Could you check a few things on this model? Use its own coordinates, in mm. A direction names the side the tool comes from. Give positions to 0.01 mm unless a question says otherwise; leave off trailing zeros. Order: outer loops, then holes, each group sorted by start corner. A loop starts at its lowest first (then second) coordinate and runs counter-clockwise, first axis right, second up.
(1) Imagine slicing it at B-B, the plane x = -42. Write out the boundary of the cut face in (y, z), then the cut area to 3 significant figures.
(2) If we mould it in two halves opening along X, with no side actions, what happens to faces 1 (the flat face through (-37.26, 20.76, -6.14)), 2 (the cylindrical face through (-44.22, 28.83, -6.03)), 3 (the flat face through (-54.102, 29, -6)), 4 (the flat face through (-44, 28, -14.719))? For each: released by +X, released by -X, zero draft, split by the parting line, or undercut.
(3) Imagine slicing it at A-A, the plane z = -4. Write out the boundary of the cut face in (x, y).
(4) Will these pins go through, and if not, where does the flat tip stop? pin 1 (7.5 mm diameter, centred on x = -45.5, y = 20.5, fed in from +Z); pin 2 (8 mm diameter, centred on y = 23, z = -11, fed in from +X); pin 3 (3 mm diameter, centred on x = -63.5, y = 9.5, fed in from -Z); pin 4 (1.5 mm diameter, centred on x = -26, z = -11, fed in from -Y).
(5) Imagine slicing it at D-D, the plane y = 7.5. Write out the boundary of the cut face in (x, z).
(6) If I drill on probe 1 along Z at (x, y) = (-51.5, 4.5); probe 2 along Y at (x, z) = (-10.5, -7.5); probe 3 along Y at (x, z) = (-52, -9), over which ranges is the centre line in solid material (lowest first)?
(7) On a 3-axis mill with a long thin cutter (end or side, diameter ignored), from which of +Z, -Z, +X, -X, +Y, -Y can I reach the whole of each face in a straight line? I mean faces 5 (the flat face through (-44, 18, -5.512)), 6 (the flat face through (-44, 18, -6.782)), 7 (the flat face through (-45, 5, -12.294)), 8 (the flat face through (-34.036, 29, -6)). Say none if no direction works.
(8) Imagine slicing it at C-C, the plane y = 15. Write out the boundary of the cut face in (x, z).
Autodesk Inventor part; units mm, degrees
ref_plane "YZ Plane" through (0, 0, 0) normal (1, 0, 0) x (0, 1, 0)
ref_plane "XZ Plane" through (0, 0, 0) normal (0, 1, 0) x (-1, 0, 0)
ref_plane "XY Plane" through (0, 0, 0) normal (0, 0, 1) x (1, 0, 0)
sketch "Sketch1" plane through (0, 0, 0) normal (0, 1, 0) x (-1, 0, 0)
  line L0 (0, 0) -> (88.138, 0)
  line L1 (88.138, 0) -> (88.138, -12.2936)
  line L2 (88.138, -12.2936) -> (0, -12.2936)
  line L3 (0, -12.2936) -> (0, 0)
  dimension "d0" = 88.138
  dimension "d1" = 12.2936
extrude "Extrusion1" add sketch "Sketch1" along normal blind 10.922
sketch "Sketch2" plane through (0, 10.922, 0) normal (0, 1, 0) x (1, 0, 0)
  line L0 (-88.138, 12.2936) -> (-88.138, 0)
  line L1 (0, 0) -> (0, 12.2936)
  line L2 (-50.038, 6.7818) -> (-38.1, 6.7818)
  line L3 (-38.1, 6.7818) -> (-38.1, 5.5118)
  line L4 (-38.1, 5.5118) -> (-50.038, 5.5118)
  line L5 (-50.038, 5.5118) -> (-50.038, 6.7818)
  dimension "d7" = 11.938
  dimension "d8" = 1.27
extrude "Extrusion2" add sketch "Sketch2" along normal blind 5.08
sketch "Sketch4" plane through (-50.038, 10.922, -5.5118) normal (0, 0, 1) x (1, 0, 0)
  line L0 (0, 5.08) -> (11.938, 5.08)
  line L1 (11.938, 5.08) -> (0, 5.08)
  line L2 (11.938, 5.08) -> (13.6399, 14.732)
  line L3 (11.938, 5.08) -> (21.7389, 5.08) construction
  line L4 (0, 5.08) -> (-1.7019, 14.732)
  line L5 (0, 5.08) -> (9.8009, 5.08) construction
  line L6 (-1.7019, 14.732) -> (13.6399, 14.732)
  point P0 (50.038, -10.922)
  dimension "d12" = 80
  dimension "d13" = 100
extrude "Extrusion3" add sketch "Sketch4" against normal blind 1.27
sketch "Sketch5" plane through (-51.7399, 25.654, -5.5118) normal (0, 1, 0) x (1, 0, 0)
  line L0 (15.3418, 0) -> (0, 0)
  line L1 (15.3418, 0) -> (15.3418, 1.27)
  line L2 (0, 1.27) -> (15.3418, 1.27)
  line L3 (0, 0) -> (0, 1.27)
  line L4 (-2.3621, 0.635) -> (17.7039, 0.635)
  line L5 (-2.3621, 9.2075) -> (17.7039, 9.2075)
  line L6 (17.7039, 9.2075) -> (17.7039, -7.9375)
  line L7 (17.7039, -7.9375) -> (-2.3621, -7.9375)
  line L8 (-2.3621, -7.9375) -> (-2.3621, 9.2075)
  point P0 (51.7399, -5.5118)
  dimension "d19" = 20.066
  dimension "d21" = 17.145
  dimension "d22" = 8.5725
  dimension "d23" = 0.635
extrude "Extrusion4" add sketch "Sketch5" along normal blind 6.35
sketch "Sketch6" plane through (-54.102, 25.654, 2.4257) normal (0, 0, 1) x (1, 0, 0)
  arc A0 (0, 6.35) -> (20.066, 6.35) centre (10.033, 20.6146) ccw
  line L0 (0, 6.35) -> (20.066, 6.35)
  point P0 (54.102, -25.654)
extrude "Extrusion5" cut sketch "Sketch6" against normal blind 20.32
properties part number "SLIDE_POTENTIOMETER"
Answer block:
1. outline: (0, -12.29) - (10.92, -12.29) - (10.92, -6.78) - (25.65, -6.78) - (25.65, -14.72) - (28.95, -14.72) - (28.95, 2.43) - (25.65, 2.43) - (25.65, -5.51) - (10.92, -5.51) - (10.92, 0) - (0, 0) - close
1. area: 210 mm2
2. face 1: released by +X
2. face 2: undercut
2. face 3: released by -X
2. face 4: zero draft
3. outline: (-88.14, 0) - (0, 0) - (0, 10.92) - (-88.14, 10.92) - close; (-54.1, 25.65) - (-34.04, 25.65) - (-34.04, 32) arc R17.44 cw to (-54.1, 32) - close
4. pin 1: stops at z = -5.51
4. pin 2: stops at x = -34.04
4. pin 3: stops at z = -12.29
4. pin 4: stops at y = 0
5. outline: (-88.14, -12.29) - (0, -12.29) - (0, 0) - (-88.14, 0) - close
6. probe 1: z = -12.29 to 0
6. probe 2: y = 0 to 10.92
6. probe 3: y = 0 to 10.92, 25.65 to 30.74
7. face 5: +Z, +X, -X
7. face 6: -Z, +X, -X
7. face 7: -Z, +X, -X, -Y
7. face 8: +Z, -Z, +X, +Y
8. outline: (-50.04, -6.78) - (-38.1, -6.78) - (-38.1, -5.51) - (-50.04, -5.51) - close
